Source: CAD feature listing. Evaluate the final solid. Frame: model axes, mm. Face numbers are marked on the shaded views. A direction names the side the tool comes from. Coordinates: 2 decimals unless noted, no trailing zeros. Order: outer loops, then holes, each group sorted by start corner. A loop starts at its lowest first (then second) coordinate and runs counter-clockwise, first axis right, second up. Notation, with made-up numbers: (49.5, 34) -> (103.5, 34) arc R21 ccw to (103.5, 63) -> close; hole circle Ø2 at (-15.5, 89). An arc over 180 degrees is marked (long way). Write item = value, one per line. Start each with the question number.
Item 1: Set-up query: the marked faces 1 and 2. Return all of +Z, -Z, +X, -X, +Y, -Y with unobstructed straight access to the full face (end or side cutting, diameter ignored); none if empty.
Item 2: Section query A-A (z = 10). Output: boundary loops of the cut face in (x, y) (1 decimal).
Item 3: Mould query, pull axis Y, two halves, no side actions, for the marked faces 3, 4, 5 and 6. Classes: released by +Y, released by -Y, zero draft, split by the parting line, or undercut.
Item 4: Contact query for flat-ended pins moving along their axis: pin 1 (14 mm diameter, centred on x = 23, y = 92.5, fed in from +Z); pin 2 (3 mm diameter, centred on y = 107.5, z = -2, fed in from -X); pin 3 (13 mm diameter, centred on x = 10, z = 0, fed in from +Y). Output: stop coordinate, or through.
Item 5: Section query D-D (z = -6.25). Output: boundary loops of the cut face in (x, y).
Item 6: Section query B-B (x = 30). Output: boundary loops of the cut face in (y, z), then the cut area to 3 significant figures.
Item 7: Ray query, line 1 along X through (y, z) = (36, 0); line 2 along Z through (x, y) = (50, 35); line 3 along Y through (x, z) = (8.5, 10). Return the intervals inside material, ascending. Write a range as [from, to].
Item 8: Section query C-C (y = 38). Output: boundary loops of the cut face in (x, z), then the cut area to 3 significant figures.
Autodesk Inventor part; units mm, degrees
ref_plane "YZ Plane" through (0, 0, 0) normal (1, 0, 0) x (0, 1, 0)
ref_plane "XZ Plane" through (0, 0, 0) normal (0, 1, 0) x (-1, 0, 0)
ref_plane "XY Plane" through (0, 0, 0) normal (0, 0, 1) x (1, 0, 0)
sketch "Boceto1" plane through (0, 0, 0) normal (0, 0, 1) x (1, 0, 0)
  point P0 (0, 0)
sketch "Boceto2" plane through (0, 0, 0) normal (0, 0, 1) x (1, 0, 0)
  line L0 (0, 0) -> (0, 100)
  line L1 (30, 130) -> (30, 130)
  line L2 (60, 100) -> (60, 0)
  line L3 (60, 0) -> (0, 0)
  arc A0 (30, 130) -> (0, 100) centre (30, 100) ccw
  arc A1 (60, 100) -> (30, 130) centre (30, 100) ccw
  point P0 (0, 130)
  point P1 (60, 130)
  dimension "d1" = 30
  dimension "d2" = 100
  dimension "d3" = 60
extrude "Extrusión1" add sketch "Boceto2" along normal mid plane 25
sketch "Boceto9" plane through (0, 0, 12.5) normal (0, -1, 0) x (1, 0, 0)
  circle A0 centre (50, -12.5) radius 4
  line L0 (60, -25) -> (0, -25)
  circle A1 centre (10, -12.5) radius 4
  line L1 (0, -12.5) -> (60, -12.5) construction
  line L2 (60, 0) -> (60, -25) construction
  line L3 (0, -25) -> (0, 0) construction
  dimension "d52" = 8
  dimension "d88" = 10
  dimension "d89" = 10
  dimension "d90" = 8
hole "Agujero4" at (10, 0, 0) at (50, 0, 0) direction (0, 1, 0) diameter 8 depth 40
thread "Rosca3"
thread "Rosca4"
sketch "Boceto10" plane through (0, 0, 12.5) normal (0, 0, 1) x (1, 0, 0)
  circle A0 centre (30, 100) radius 13
  circle A1 centre (30, 100) radius 23.5125
  line L0 (60, 0) -> (60, 100)
  line L1 (0, 100) -> (0, 0)
  line L2 (40, 144.843) -> (20, 144.843)
  dimension "d64" = 26
  dimension "d65" = 30
  dimension "d68" = 47.025
  dimension "d91" = 100
extrude "Extrusión5" cut sketch "Boceto10" against normal through all contours A0
extrude "Extrusión6" cut sketch "Boceto10" against normal blind 13
sketch "Boceto12" plane through (0, 0, 12.5) normal (0, 0, 1) x (1, 0, 0)
  line L0 (6, 40) -> (14, 40) construction
  line L1 (10, 40) -> (10, 0) construction
  line L2 (46, 40) -> (54, 40) construction
  line L3 (50, 40) -> (50, 0) construction
  line L4 (0, 0) -> (60, 0) construction
  line L5 (3.4875, 21.5) -> (16.5125, 21.5)
  line L6 (16.5125, 21.5) -> (16.5125, 15)
  line L7 (16.5125, 15) -> (3.4875, 15)
  line L8 (3.4875, 15) -> (3.4875, 21.5)
  line L9 (43.4875, 21.5) -> (56.5125, 21.5)
  line L10 (43.4875, 15) -> (43.4875, 21.5)
  line L11 (56.5125, 15) -> (43.4875, 15)
  line L12 (56.5125, 21.5) -> (56.5125, 15)
  dimension "d92" = 13.025
  dimension "d93" = 6.5125
  dimension "d94" = 15
  dimension "d95" = 6.5
  dimension "d98" = 40
extrude "Extrusión7" cut sketch "Boceto12" against normal blind 23.0125
properties part number "soporte_riel" material "Nilón 6/6"
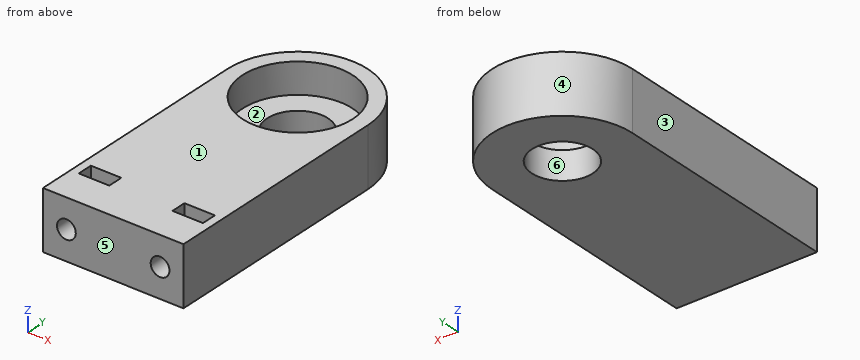
Computed:
q1.face_1 = +Z, +X, -X, +Y, -Y
q1.face_2 = +Z
q2.outline = (0, 0) -> (60, 0) -> (60, 100) arc R30 ccw to (0, 100) -> close; hole (3.5, 15) -> (16.5, 15) -> (16.5, 21.5) -> (3.5, 21.5) -> close; hole circle Ø47 at (30, 100); hole (43.5, 15) -> (56.5, 15) -> (56.5, 21.5) -> (43.5, 21.5) -> close
q3.face_3 = zero draft
q3.face_4 = released by +Y
q3.face_5 = released by -Y
q3.face_6 = undercut
q4.pin_1 = -0.5
q4.pin_2 = 0.61
q4.pin_3 = 126.79
q5.outline = (0, 0) -> (60, 0) -> (60, 100) arc R30 ccw to (0, 100) -> close; hole (3.49, 15) -> (16.51, 15) -> (16.51, 21.5) -> (3.49, 21.5) -> close; hole circle Ø26 at (30, 100); hole (43.49, 15) -> (56.51, 15) -> (56.51, 21.5) -> (43.49, 21.5) -> close
q6.outline = (0, -12.5) -> (87, -12.5) -> (87, -0.5) -> (76.49, -0.5) -> (76.49, 12.5) -> (0, 12.5) -> close; (113, -12.5) -> (130, -12.5) -> (130, 12.5) -> (123.51, 12.5) -> (123.51, -0.5) -> (113, -0.5) -> close
q6.area = 2,330 mm^2
q7.line_1 = [0, 6], [14, 46], [54, 60]
q7.line_2 = [-12.5, -4], [4, 12.5]
q7.line_3 = [0, 15], [21.5, 90.48], [109.52, 120.92]
q8.outline = (0, -12.5) -> (60, -12.5) -> (60, 12.5) -> (0, 12.5) -> close; hole circle Ø8 at (10, 0); hole circle Ø8 at (50, 0)
q8.area = 1,400 mm^2
